```python
from build123d import *

# Parameters (mm, degrees)
SKETCH1_R               = 7.5
BOSS_EXTRUDE1_DEPTH     = 35.4
SKETCH3_W               = 10
SKETCH3_H               = 16
CUT_EXTRUDE2_DEPTH      = 10
CUT_EXTRUDE3_DEPTH      = 37.954837302
CUT_EXTRUDE3_DEPTH_BACK = 37.954837302
CUT_EXTRUDE4_DEPTH      = 37.954837438
CUT_EXTRUDE4_DEPTH_BACK = 37.954837438
SKETCH5_R               = 1.5
FILLET1_R               = 0.1
SKETCH6_W               = 20
SKETCH6_H               = 20
BOSS_EXTRUDE2_DEPTH     = 3


with BuildPart() as part:
    # Sketch1 → Boss-Extrude1 (new body)
    with BuildSketch(Plane.XY):
        Circle(SKETCH1_R)
    extrude(amount=BOSS_EXTRUDE1_DEPTH)

    # Sketch3 → Cut-Extrude2 (cut)
    with BuildSketch(Plane.XY.offset(35.4)):
        Rectangle(SKETCH3_W, SKETCH3_H)
    extrude(amount=-CUT_EXTRUDE2_DEPTH, mode=Mode.SUBTRACT)

    # Sketch4 → Cut-Extrude3 (cut, two sides: drawn at the far end of the back side and taken through both)
    with BuildSketch(Plane(origin=(0, 0, 0), x_dir=(0, 0, -1), z_dir=(1, 0, 0)).offset(-CUT_EXTRUDE3_DEPTH_BACK)):
        with BuildLine():
            Line((-25.4, 76.496949074), (-25.4, 7.5))
            Line((-25.4, 7.5), (-25.4, 5.590169944))
            Line((-25.4, 5.590169944), (-32.352923855, 3.884664175))
            ThreePointArc((-32.352923855, 3.884664175), (-35.399999999, -0.000262165), (-32.352744721, -3.885047998))
            Line((-32.352744721, -3.885047998), (-25.4, -5.590169944))
            Line((-25.4, -5.590169944), (-25.4, -7.5))
            Line((-25.4, -7.5), (-25.4, -76.496949074))
            Line((-25.4, -76.496949074), (-163.393898147, -76.496949074))
            Line((-163.393898147, -76.496949074), (-163.393898147, 76.496949074))
            Line((-163.393898147, 76.496949074), (-25.4, 76.496949074))
        make_face()
    extrude(amount=CUT_EXTRUDE3_DEPTH + CUT_EXTRUDE3_DEPTH_BACK, mode=Mode.SUBTRACT)

    # Sketch5 → Cut-Extrude4 (cut, two sides: drawn at the far end of the back side and taken through both)
    with BuildSketch(Plane(origin=(0, 0, 0), x_dir=(0, 0, -1), z_dir=(1, 0, 0)).offset(-CUT_EXTRUDE4_DEPTH_BACK)):
        with Locations(Location((-31.4, -0.000169944, 0), (0, 0, 0.006491373))):
            Circle(SKETCH5_R)
    extrude(amount=CUT_EXTRUDE4_DEPTH + CUT_EXTRUDE4_DEPTH_BACK, mode=Mode.SUBTRACT)

    # Fillet1
    # the kernel refuses this fillet: 0.1 mm, written as the material it takes off along each edge
    with BuildSketch(Plane(origin=(0, 0, 25.4), x_dir=(0.6911452834399253, -0.7227158481580055, 0), z_dir=(0.7227158481580055, 0.6911452834399253, 0))) as fillet1_piece_1_section:
        with BuildLine():
            CenterArc((7.5 - FILLET1_R, FILLET1_R), FILLET1_R, 270, 90)
            Line((7.5 - FILLET1_R, 0), (7.5, 0))
            Line((7.5, 0), (7.5, FILLET1_R))
        make_face()
    fillet1_piece_1 = revolve(axis=Axis((0, 0, 25.4), (0, 0, -1)), revolution_arc=87.441672972, mode=Mode.PRIVATE)
    fillet1_piece_1 = split(fillet1_piece_1, bisect_by=Plane(origin=(5, -5.569278589, 25.383070115), z_dir=(-1, 0, 0)), keep=Keep.TOP, mode=Mode.PRIVATE)
    fillet1_piece_1 = split(fillet1_piece_1, bisect_by=Plane(origin=(-5, -5.569278589, 25.383070115), z_dir=(1, 0, 0)), keep=Keep.TOP, mode=Mode.PRIVATE)
    add(fillet1_piece_1, mode=Mode.SUBTRACT)
    with BuildSketch(Plane(origin=(0, 0, 25.4), x_dir=(-0.6911452834399255, 0.7227158481580054, 0), z_dir=(-0.7227158481580054, -0.6911452834399255, 0))) as fillet1_piece_2_section:
        with BuildLine():
            CenterArc((7.5 - FILLET1_R, FILLET1_R), FILLET1_R, 270, 90)
            Line((7.5 - FILLET1_R, 0), (7.5, 0))
            Line((7.5, 0), (7.5, FILLET1_R))
        make_face()
    fillet1_piece_2 = revolve(axis=Axis((0, 0, 25.4), (0, 0, -1)), revolution_arc=87.441672972, mode=Mode.PRIVATE)
    fillet1_piece_2 = split(fillet1_piece_2, bisect_by=Plane(origin=(5, 5.569279486, 25.383069507), z_dir=(-1, 0, 0)), keep=Keep.TOP, mode=Mode.PRIVATE)
    fillet1_piece_2 = split(fillet1_piece_2, bisect_by=Plane(origin=(-5, 5.569279486, 25.383069507), z_dir=(1, 0, 0)), keep=Keep.TOP, mode=Mode.PRIVATE)
    add(fillet1_piece_2, mode=Mode.SUBTRACT)

    # Sketch6 → Boss-Extrude2 (add)
    with BuildSketch(Plane(origin=(0, 0, 0), x_dir=(-1, 0, 0), z_dir=(0, 0, -1))):
        Rectangle(SKETCH6_W, SKETCH6_H)
    extrude(amount=BOSS_EXTRUDE2_DEPTH)


solid = part.part
```
The listing builds one solid part. Answer for the finished solid, in the listing's coordinates (mm). A direction names the side the tool comes from. Give positions to 0.01 mm unless a question says otherwise; leave off trailing zeros. Loops run counter-clockwise (first coordinate to the right, second up) from the corner with the lowest first, then second, coordinate; pieces in that order, holes last. Notation, with made-up numbers: (4.5, -34) - (13.5, -34) arc R18 cw to (13.5, -28) - close; hole circle Ø11 at (26.5, 15). An arc over 180 degrees is marked (long way). Return JSON: item names as keys, results as strings. Group by question number.
1. Given pin 1 Ø2 at (x, z) = (6.5, 22.5) entering from +Y; pin 2 Ø5 at (x, y) = (-0.5, 3.5) entering from +Z; pin 3 Ø12 at (y, z) = (-4, 9) entering from -X; pin 4 Ø2.5 at (y, z) = (0, 31.4) entering from -X (3 decimals), each flat-ended and moving along its own axis, determine where each tip first touches the part or whether it passes through.
2. Find section C-C (x = 0). Write down the section's boundary in (y, z).
3. Find section B-B (z = 31.4). Write down the section's boundary in (x, y), then the cut area to 3 significant figures.
4. Straight lines are drawn through the part: line 1 (X direction, y = 0.25, z = 26); line 2 (X direction, y = 0.25, z = 24.5); line 3 (Z direction, x = -2, y = -0.75). For each, find the intervals that lie inside material, in ascending order. Write a range as [from, to].
5. Which of the six approach directions +Z, -Z, +X, -X, +Y, -Y give full straight-line access (tool end or side, diameter ignored) to faces 1 (the cylindrical face through (3.461, -6.654, 13.519)), 2 (the cylindrical face through (-6.269, 1.487, 31.595)), 3 (the flat face through (0, 0, 25.4))?
6. Find section D-D (z = 5.5). Write down the section's boundary in (x, y).
7. Find section A-A (y = 0). Write down the section's boundary in (x, z), then the cut area to 3 significant figures.
8. Determine the mould class of faces 4 (the flat face through (0, -10, -1)), 5 (the cylindrical face through (6, 0.1, 35.4)), 6 (the cylindrical face through (6.23, 0.07, 32.9)) for opening direction Y: pulls with the +Y half, pulls with the -Y half, needs draft (parallel to the pull), parting line crosses it, or undercut.
Verdict:
{
 "1": {"pin 1": "stops at y = 5.1", "pin 2": "stops at z = 25.4", "pin 3": "stops at x = -7.5", "pin 4": "passes through"},
 "2": {"outline": "(-10, -3) - (10, -3) - (10, 0) - (7.5, 0) - (7.5, 25.3) arc R0.1 ccw to (7.4, 25.4) - (-7.4, 25.4) arc R0.1 ccw to (-7.5, 25.3) - (-7.5, 0) - (-10, 0) - close"},
 "3": {"outline": "(-7.35, -1.5) arc R7.5 ccw to (-6.27, -4.12) - (-5, -4.12) - (-5, -1.5) - close; (-7.35, 1.5) - (-5, 1.5) - (-5, 4.12) - (-6.27, 4.12) arc R7.5 ccw to start; (5, -4.12) - (6.27, -4.12) arc R7.5 ccw to (7.35, -1.5) - (5, -1.5) - close; (5, 1.5) - (7.35, 1.5) arc R7.5 ccw to (6.27, 4.12) - (5, 4.12) - close", "area": "20.0 mm^2"},
 "4": {"line 1": "x = [-7.5, -5], [5, 7.5]", "line 2": "x = [-7.5, 7.5]", "line 3": "z = [-3, 25.4]"},
 "5": {"face 1": "+Z", "face 2": "+X, -X", "face 3": "+Z, +Y, -Y"},
 "6": {"outline": "circle Ø15 at (0, 0)"},
 "7": {"outline": "(-10, -3) - (10, -3) - (10, 0) - (7.5, 0) - (7.5, 29.9) - (5, 29.9) - (5, 25.4) - (-5, 25.4) - (-5, 29.9) - (-7.5, 29.9) - (-7.5, 0) - (-10, 0) - close; (-7.5, 32.9) - (-5, 32.9) - (-5, 35.4) - (-7.5, 35.4) - close; (5, 32.9) - (7.5, 32.9) - (7.5, 35.4) - (5, 35.4) - close", "area": "476 mm^2"},
 "8": {"face 4": "pulls with the -Y half", "face 5": "parting line crosses it", "face 6": "undercut"}
}
